```python
from build123d import *

# Parameters (mm, degrees)
SKETCH003_W        = 71
SKETCH003_H        = 71
PAD001_DEPTH       = 3
SKETCH004_W        = 71
SKETCH004_H        = 71
SKETCH004_W_2      = 65
SKETCH004_H_2      = 65
PAD002_DEPTH       = 30
SKETCH005_W        = 7.5
SKETCH005_H        = 7.5
PAD003_DEPTH       = 23
SKETCH006_R        = 1.3
POCKET002_DEPTH    = 16
POCKET003_DEPTH    = 0.2
POCKET004_DEPTH    = 0.2
POCKET005_DEPTH    = 0.2
POCKET005_FACE10_W = 65.4
POCKET005_FACE10_H = 30
POCKET006_DEPTH    = 0.2
SKETCH009_W        = 14
SKETCH009_H        = 2.5
SKETCH009_H_2      = 13
POCKET012_DEPTH    = 5
CHAMFER001_SIZE    = 2
SKETCH010_R        = 6.25
POCKET013_DEPTH    = 5
SKETCH011_W        = 5
SKETCH011_H        = 10
SKETCH011_H_2      = 6
POCKET014_DEPTH    = 5
CHAMFER003_SIZE    = 2
SKETCH012_R        = 2
POCKET015_DEPTH    = 5


with BuildPart() as part:
    # Sketch003 → Pad001 (new body)
    with BuildSketch(Plane.XY):
        Rectangle(SKETCH003_W, SKETCH003_H)
    extrude(amount=PAD001_DEPTH)

    # Sketch004 (on Face6 of Pad001) → Pad002 (join)
    with BuildSketch(Plane.XY.offset(3)):
        Rectangle(SKETCH004_W, SKETCH004_H)
        Rectangle(SKETCH004_W_2, SKETCH004_H_2, mode=Mode.SUBTRACT)
    extrude(amount=PAD002_DEPTH)

    # Sketch005 (on Face15 of Pad002) → Pad003 (join)
    with BuildSketch(Plane.XY.offset(3)):
        with Locations((-28.75, 28.75)):
            Rectangle(SKETCH005_W, SKETCH005_H)
        with Locations((28.75, 28.75)):
            Rectangle(SKETCH005_W, SKETCH005_H)
        with Locations((28.75, -11.5)):
            Rectangle(SKETCH005_W, SKETCH005_H)
        with Locations((-28.75, -11.5)):
            Rectangle(SKETCH005_W, SKETCH005_H)
    extrude(amount=PAD003_DEPTH)

    # Sketch006 (on Face20 of Pad003) → Pocket002 (cut)
    with BuildSketch(Plane.XY.offset(26)):
        with Locations((-28.5, 28.5)):
            Circle(SKETCH006_R)
        with Locations((28.5, 28.5)):
            Circle(SKETCH006_R)
        with Locations((28.5, -11.5)):
            Circle(SKETCH006_R)
        with Locations((-28.5, -11.5)):
            Circle(SKETCH006_R)
    extrude(amount=-POCKET002_DEPTH, mode=Mode.SUBTRACT)

    # Pocket002 Face11 → Pocket003 (cut)
    with BuildSketch(Plane(origin=(-32.5, -1.853972, 18.752336), x_dir=(0, -1, 0), z_dir=(1, 0, 0))):
        Polygon((30.646028, 15.752336), (13.396028, 15.752336), (13.396028, -7.247664), (5.896028, -7.247664), (5.896028, 15.752336), (-26.853972, 15.752336), (-26.853972, -7.247664), (-34.353972, -7.247664), (-34.353972, -14.247664), (30.646028, -14.247664), align=None)
    extrude(amount=-POCKET003_DEPTH, mode=Mode.SUBTRACT)

    # Pocket003 Face15 → Pocket004 (cut)
    with BuildSketch(Plane(origin=(32.5, -1.853972, 18.752336), x_dir=(0, 1, 0), z_dir=(-1, 0, 0))):
        Polygon((34.353972, -7.247664), (26.853972, -7.247664), (26.853972, 15.752336), (-5.896028, 15.752336), (-5.896028, -7.247664), (-13.396028, -7.247664), (-13.396028, 15.752336), (-30.646028, 15.752336), (-30.646028, -14.247664), (34.353972, -14.247664), align=None)
    extrude(amount=-POCKET004_DEPTH, mode=Mode.SUBTRACT)

    # Pocket004 Face2 → Pocket005 (cut)
    with BuildSketch(Plane(origin=(0, 32.5, 18.771054), x_dir=(-1, 0, 0), z_dir=(0, -1, 0))):
        Polygon((32.7, -7.228946), (25, -7.228946), (25, 15.771054), (-25, 15.771054), (-25, -7.228946), (-32.7, -7.228946), (-32.7, -14.228946), (32.7, -14.228946), align=None)
    extrude(amount=-POCKET005_DEPTH, mode=Mode.SUBTRACT)

    # Pocket005 Face10 → Pocket006 (cut)
    with BuildSketch(Plane(origin=(0, -32.5, 18), x_dir=(1, 0, 0), z_dir=(0, 1, 0))):
        Rectangle(POCKET005_FACE10_W, POCKET005_FACE10_H)
    extrude(amount=-POCKET006_DEPTH, mode=Mode.SUBTRACT)

    # Sketch009 (on Face17 of Pocket006) → Pocket012 (cut)
    with BuildSketch(Plane.XZ.offset(35.5)):
        with Locations((-24.25, 25.25)):
            Rectangle(SKETCH009_W, SKETCH009_H)
        with Locations((23.75, 20.25)):
            Rectangle(SKETCH009_W, SKETCH009_H_2)
    extrude(amount=-POCKET012_DEPTH, mode=Mode.SUBTRACT)

    # Chamfer001
    chamfer001_edges = [part.edges().sort_by_distance(p)[0] for p in [
        (-24.25, -35.5, 24),
        (-24.25, -35.5, 26.5),
    ]]
    chamfer(chamfer001_edges, length=CHAMFER001_SIZE)

    # Sketch010 (on Face33 of Chamfer001) → Pocket013 (cut)
    with BuildSketch(Plane(origin=(0, 35.5, 0), x_dir=(-1, 0, 0), z_dir=(0, 1, 0))):
        with Locations((-18.6, 11.5)):
            Circle(SKETCH010_R)
    extrude(amount=-POCKET013_DEPTH, mode=Mode.SUBTRACT)

    # Sketch011 (on Face18 of Pocket013) → Pocket014 (cut)
    with BuildSketch(Plane(origin=(0, 0, 0), x_dir=(1, 0, 0), z_dir=(0, 0, -1))):
        with Locations((28.75, -19.25)):
            Rectangle(SKETCH011_W, SKETCH011_H)
        with Locations((28.75, -5.25)):
            Rectangle(SKETCH011_W, SKETCH011_H_2)
    extrude(amount=-POCKET014_DEPTH, mode=Mode.SUBTRACT)

    # Chamfer003
    chamfer003_edges = [part.edges().sort_by_distance(p)[0] for p in [
        (0, 35.5, 0),
        (35.5, 0, 0),
        (0, -35.5, 0),
        (-35.5, 0, 0),
    ]]
    chamfer(chamfer003_edges, length=CHAMFER003_SIZE)

    # Sketch012 (on Face1 of Chamfer003) → Pocket015 (cut)
    with BuildSketch(Plane.XZ.offset(35.5)):
        with Locations((-10.25, 21)):
            Circle(SKETCH012_R)
        with Locations((9.75, 21)):
            Circle(SKETCH012_R)
        with Locations((-10.25, 11)):
            Circle(SKETCH012_R)
        with Locations((9.75, 11)):
            Circle(SKETCH012_R)
    extrude(amount=-POCKET015_DEPTH, mode=Mode.SUBTRACT)


with BuildPart() as part_1:
    # Body001 placement: moved
    add(part.part.moved(Location((0, 0, -25.94))))


solid = part_1.part
```
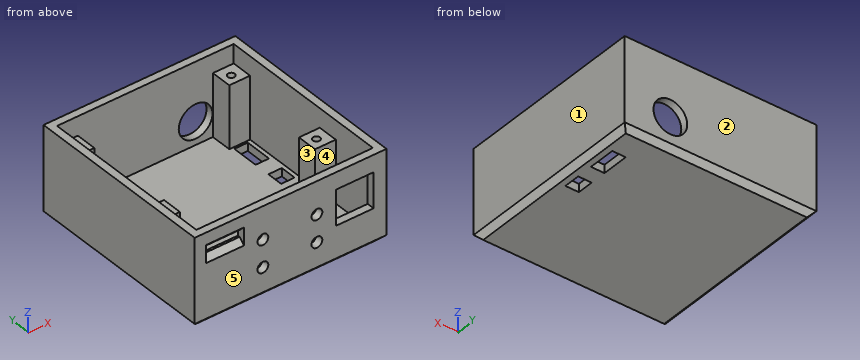
Check sheet for the modelled part. Datum: model origin and axes. Units: mm. Face numbers are marked on the shaded views. A direction names the side the tool comes from. Round coordinates to 2 decimals unless told otherwise and drop trailing zeros. Write each loop counter-clockwise with the first axis right and the second up, starting at its lowest first coordinate (ties: lowest second). Pieces come first, ordered by that corner, then holes. Notation, with made-up numbers: (19, 14) -> (28, 14) arc R26 ccw to (28, 28) -> close; hole circle Ø6 at (56, 25). An arc over 180 degrees is marked (long way). Put each result on its own line as item: value.
(1) Material ranges on line 1 (Y direction, x = -27, z = -9); line 2 (Y direction, x = -10, z = -0.5), recorded low to high.
Values found:
line 1: y = -35.5 to -32.7, -15.25 to -7.75, 25 to 35.5
line 2: y = -35.5 to -32.7, 32.7 to 35.5
(2) Tool access check on the marked faces 4 and 5. Record the directions out of +Z, -Z, +X, -X, +Y, -Y that give a thin tool (end or side, any length) a straight path to the whole face; none if there is none.
Values found:
face 4: +Z
face 5: +Z, -Z, +X, -X, -Y
(3) Sectioned sample at A-A (x = -23). Enter the section's corners in (y, z).
Values found:
outline: (-35.5, -23.94) -> (-33.5, -25.94) -> (33.5, -25.94) -> (35.5, -23.94) -> (35.5, 7.06) -> (32.7, 7.06) -> (32.7, -22.94) -> (-32.7, -22.94) -> (-32.7, -1.94) -> (-33.5, -1.94) -> (-35.5, -3.94) -> close; (-35.5, 2.56) -> (-33.5, 0.56) -> (-32.7, 0.56) -> (-32.7, 7.06) -> (-35.5, 7.06) -> close
(4) Go/stop test with flat-tipped pins: pin 1 Ø1.6 at (x, y) = (28.5, -11.5) entering from +Z; pin 2 Ø2.5 at (x, y) = (-30, 30.5) entering from +Z; pin 3 Ø4 at (x, z) = (28, -9) entering from -Y. Record where each tip stops, or that it passes through.
Values found:
pin 1: stops at z = -15.94
pin 2: stops at z = 0.06
pin 3: stops at y = -15.25
(5) Sectioned sample at C-C (y = 19). Enter the section's corners in (x, z), plus the area to 3 significant figures.
Values found:
outline: (-35.5, -23.94) -> (-33.5, -25.94) -> (26.25, -25.94) -> (26.25, -22.94) -> (-32.7, -22.94) -> (-32.7, 7.06) -> (-35.5, 7.06) -> close; (31.25, -25.94) -> (33.5, -25.94) -> (35.5, -23.94) -> (35.5, 7.06) -> (32.7, 7.06) -> (32.7, -22.94) -> (31.25, -22.94) -> close
area: 362 mm^2
(6) Mould release check, pull along Y, two halves, no side actions. Record for the marked faces 1, 2 and 3: released by +Y, released by -Y, zero draft, split by the parting line, or undercut.
Values found:
face 1: zero draft
face 2: released by +Y
face 3: undercut
(7) Sectioned sample at B-B (z = -22). Enter the section's corners in (x, y), plus the area to 3 significant figures.
Values found:
outline: (-35.5, -35.5) -> (35.5, -35.5) -> (35.5, 35.5) -> (-35.5, 35.5) -> close; hole (-32.7, -32.7) -> (32.7, -32.7) -> (32.7, -15.25) -> (25, -15.25) -> (25, -7.75) -> (32.7, -7.75) -> (32.7, 25) -> (25, 25) -> (25, 32.7) -> (-25, 32.7) -> (-25, 25) -> (-32.7, 25) -> (-32.7, -7.75) -> (-25, -7.75) -> (-25, -15.25) -> (-32.7, -15.25) -> close
area: 998 mm^2
(8) Sectioned sample at D-D (x = 18.6). Enter the section's corners in (y, z).
Values found:
outline: (-35.5, -23.94) -> (-33.5, -25.94) -> (33.5, -25.94) -> (35.5, -23.94) -> (35.5, -20.69) -> (32.7, -20.69) -> (32.7, -22.94) -> (-32.7, -22.94) -> (-32.7, -12.19) -> (-35.5, -12.19) -> close; (-35.5, 0.81) -> (-32.7, 0.81) -> (-32.7, 7.06) -> (-35.5, 7.06) -> close; (32.7, -8.19) -> (35.5, -8.19) -> (35.5, 7.06) -> (32.7, 7.06) -> close
